```python
from build123d import *

# Parameters (mm, degrees)
SKETCH1_W               = 59.436
SKETCH1_H               = 17.399
BOSS_EXTRUDE1_DEPTH     = 2.54
CUT_EXTRUDE1_DEPTH      = 32.069155512
SKETCH3_W               = 12.7
SKETCH3_H               = 6.35
BOSS_EXTRUDE2_DEPTH     = 2.032
BOSS_EXTRUDE3_DEPTH     = 15.24
CUT_EXTRUDE2_DEPTH      = 47.886984472
CUT_EXTRUDE2_DEPTH_BACK = 47.886984472
RIB1_REACH              = 48.887
SKETCH6_WALL_W          = 104.28296917
SKETCH6_WALL_H          = 5.08


with BuildPart() as part:
    # Sketch1 → Boss-Extrude1 (new body)
    with BuildSketch(Plane(origin=(0, 0, 0), x_dir=(1, 0, 0), z_dir=(0, 1, 0))):
        Rectangle(SKETCH1_W, SKETCH1_H)
    extrude(amount=BOSS_EXTRUDE1_DEPTH)

    # Sketch2 → Cut-Extrude1 (cut, through all)
    with BuildSketch(Plane(origin=(0, 2.54, 0), x_dir=(1, 0, 0), z_dir=(0, 1, 0))):
        with BuildLine():
            Line((-29.718, 0), (-29.718, 4.445))
            Line((-29.718, 4.445), (-10.668, 4.445))
            ThreePointArc((-10.668, 4.445), (-6.223, 0), (-10.668, -4.445))
            Line((-10.668, -4.445), (-29.718, -4.445))
            Line((-29.718, -4.445), (-29.718, 0))
        make_face()
    extrude(amount=-CUT_EXTRUDE1_DEPTH, mode=Mode.SUBTRACT)

    # Sketch3 → Boss-Extrude2 (add)
    with BuildSketch(Plane.XY.offset(8.6995)):
        with Locations((-29.718, 3.175)):
            Rectangle(SKETCH3_W, SKETCH3_H)
    boss_extrude2 = extrude(amount=BOSS_EXTRUDE2_DEPTH)

    # Mirror1: Boss-Extrude2 across plane
    add(boss_extrude2.mirror(Plane.XY))

    # Sketch4 → Boss-Extrude3 (add)
    with BuildSketch(Plane(origin=(29.718, 0, 0), x_dir=(0, 0, -1), z_dir=(1, 0, 0))):
        with BuildLine():
            Line((-5.3594, 7.874163869), (5.3594, 7.874163869))
            ThreePointArc((5.3594, 7.874163869), (9.395879403, 1.563033987), (7.62, -5.715))
            Line((7.62, -5.715), (-7.62, -5.715))
            ThreePointArc((-7.62, -5.715), (-9.395879403, 1.563033987), (-5.3594, 7.874163869))
        make_face()
    extrude(amount=BOSS_EXTRUDE3_DEPTH)

    # Sketch5 → Cut-Extrude2 (cut, two sides)
    with BuildSketch(Plane.XY) as cut_extrude2_sk:
        with BuildLine():
            Line((-125.410978847, 85.578603758), (30.353, 7.874163869))
            ThreePointArc((30.353, 7.874163869), (38.487292522, 2.407660331), (44.958, -4.953))
            Line((44.958, -4.953), (142.117632376, -149.38430866))
            Line((142.117632376, -149.38430866), (371.853916425, 112.19326708))
            Line((371.853916425, 112.19326708), (104.325305202, 347.156179498))
            Line((104.325305202, 347.156179498), (-125.410978847, 85.578603758))
        make_face()
    extrude(amount=CUT_EXTRUDE2_DEPTH, mode=Mode.SUBTRACT)
    extrude(cut_extrude2_sk.sketch, amount=-CUT_EXTRUDE2_DEPTH_BACK, mode=Mode.SUBTRACT)

    # Sketch6 wall → Rib1 (add, up to next)
    with BuildSketch(Plane(origin=(25.908, 4.433322543, 0), x_dir=(0.895522388061, 0.445016463157, 0), z_dir=(-0.445016463157, 0.895522388061, 0)), mode=Mode.PRIVATE) as rib1_sk1:
        Rectangle(SKETCH6_WALL_W, SKETCH6_WALL_H)
    rib1_tool1 = extrude(rib1_sk1.sketch, amount=-RIB1_REACH, mode=Mode.PRIVATE) - part.part
    add(rib1_tool1.solids().sort_by_distance((25.908, 4.433322543, 0))[0])


solid = part.part
```
Check sheet for the modelled part. Datum: model origin and axes. Units: mm. A direction names the side the tool comes from. Round coordinates to 2 decimals unless told otherwise and drop trailing zeros. Loops run counter-clockwise (first coordinate to the right, second up) from the corner with the lowest first, then second, coordinate; pieces in that order, holes last. Notation, with made-up numbers: (-30.75, 61) -> (12.25, 61) arc R22 cw to (12.25, 78) -> close; hole circle Ø4 at (62, 21.5). An arc over 180 degrees is marked (long way). Write item = value, one per line. Start each with the question number.
1) Gauge pin test, flat ends, axial feed: pin 1 Ø3 at (x, z) = (-5, 7.5) entering from +Y; pin 2 Ø1.1 at (x, y) = (25.5, 4.5) entering from -Z; pin 3 Ø1.6 at (x, z) = (-31, 9.5) entering from +Y. Record the tip position at first contact, or that the pin passes through.
2) Release check for a two-part mould opening along Z. For faces 1 (the flat face through (-23.368, 3, 10)), 2 (the flat face through (-20, 1, -4.445)), 3 (the cylindrical face through (35.538, -0.033, -9.525)), 4 (the flat face through (3, 1, 8.7)) record: released by +Z, released by -Z, zero draft, split by the parting line, or undercut.
3) Sectioned sample at B-B, the plane z = 0. Record the cut outline in (x, y) (3 decimals).
4) Sectioned sample at D-D, the plane x = 24. Record the cut outline in (y, z), plus the area to 3 significant figures.
5) Thickness scan on probe 1 along Z at (x, y) = (-27, 3.25); probe 2 along Z at (x, y) = (27.5, 4); probe 3 along Y at (x, z) = (-9.5, 6.75). Record the ranges inside material, lowest first.
6) Set-up check for faces 5 (the flat face through (27, 4, -2.54)), 6 (the flat face through (-31, 4, 8.7)), 7 (the flat face through (3, 1, -8.7)), 8 (the flat face through (27, 4, 2.54)), 9 (the cylindrical face through (35.54, -0.25, 9.52)): record each of +Z, -Z, +X, -X, +Y, -Y from which the full face is reachable in a straight line by a thin tool's end or side.
7) Sectioned sample at C-C, the plane y = 3.25. Record the cut outline in (x, z).
Results are:
q1.pin_1 = 2.54
q1.pin_2 = -2.54
q1.pin_3 = 6.35
q2.face_1 = zero draft
q2.face_2 = undercut
q2.face_3 = released by -Z
q2.face_4 = released by +Z
q3.outline = (-6.223, 0) -> (29.718, 0) -> (29.718, -5.715) -> (44.958, -5.715) -> (44.958, -4.953) arc R38.1 ccw to (30.353, 7.874) -> (29.718, 7.874) -> (29.718, 6.327) -> (22.098, 2.54) -> (-6.223, 2.54) -> close
q4.outline = (0, -8.7) -> (2.54, -8.7) -> (2.54, -2.54) -> (3.49, -2.54) -> (3.49, 2.54) -> (2.54, 2.54) -> (2.54, 8.7) -> (0, 8.7) -> close
q4.area = 49.0 mm^2
q5.probe_1 = -10.73 to -8.7, 8.7 to 10.73
q5.probe_2 = -2.54 to 2.54
q5.probe_3 = 0 to 2.54
q6.face_5 = -Z, -X, +Y
q6.face_6 = -X, +Y
q6.face_7 = -Z, +Y, -Y
q6.face_8 = +Z, -X, +Y
q6.face_9 = +Z, +X
q7.outline = (-36.07, -10.73) -> (-23.37, -10.73) -> (-23.37, -8.7) -> (-36.07, -8.7) -> close; (-36.07, 8.7) -> (-23.37, 8.7) -> (-23.37, 10.73) -> (-36.07, 10.73) -> close; (23.53, -2.54) -> (29.72, -2.54) -> (29.72, -8.95) -> (37.49, -8.95) -> (37.49, 8.95) -> (29.72, 8.95) -> (29.72, 2.54) -> (23.53, 2.54) -> close
